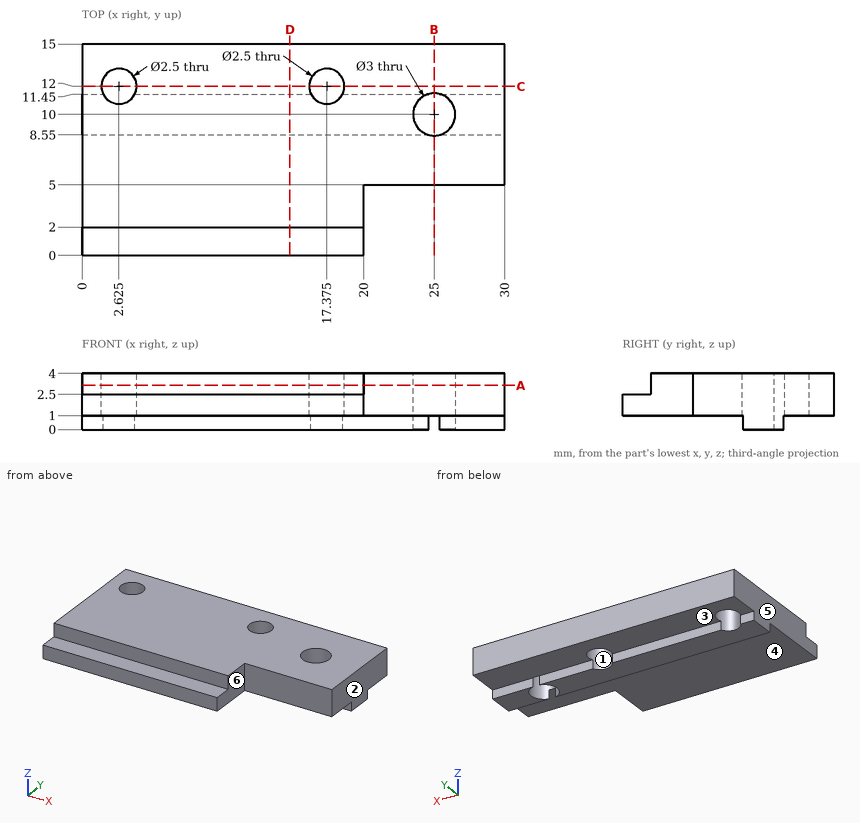
For this review, use the dimensioned drawing (mm, ordinates from the lowest corner) and the shaded views. A direction names the side the tool comes from. Give positions to 0.01 mm unless a question says otherwise; leave off trailing zeros. Loops run counter-clockwise (first coordinate to the right, second up) from the corner with the lowest first, then second, coordinate; pieces in that order, holes last.
Item 1: Insertion check: pin 1 (0.5 mm diameter, centred on x = 7.5, z = 0.5, fed in from +Y); pin 2 (0.8 mm diameter, centred on x = 1, z = 0.5, fed in from +Y); pin 3 (0.5 mm diameter, centred on x = 16.5, z = 0.5, fed in from -Y). Each pin has a flat end and moves straight along its axis. Give the tip position at first contact, or say it passes through.
Item 2: For line 1 along X through (y, z) = (12, 3.1) (3 decimals); line 2 along Y through (x, z) = (25, 2.15); line 3 along X through (y, z) = (10, 0.9), list the stretches that pass through material, from the lowest coordinate up.
Item 3: Take a section at B-B, the plane x = 25. State the section outline as (y, z) points.
Item 4: Take a section at C-C, the plane y = 12. State the section outline as (x, z) points (3 decimals).
Item 5: Take a section at A-A, the plane z = 3.15. State the section outline as (x, y) points (3 decimals).
Item 6: Tool access review of the marked faces 4, 5 and 6: name each direction out of +Z, -Z, +X, -X, +Y, -Y from which nothing blocks a thin tool from reaching the whole face with its end or side.
Item 7: Draft analysis for pull direction X (two halves, no side actions). For the marked faces 1, 2 and 3, state which applies: +X half, -X half, draft (parallel to the pull), parting line (faces both ways), or undercut.
Item 8: Take a section at D-D, the plane x = 14.75. State the section outline as (y, z) points, and give its area (3 significant figures).
Calculated:
1. pin 1: stops at y = 11.45
1. pin 2: stops at y = 11.45
1. pin 3: stops at y = 8.55
2. line 1: x = 0 to 1.375, 3.875 to 16.125, 18.625 to 30
2. line 2: y = 5 to 8.5, 11.5 to 15
2. line 3: x = 0 to 23.5, 26.5 to 30
3. outline: (5, 1) - (8.5, 1) - (8.5, 4) - (5, 4) - close; (11.5, 1) - (15, 1) - (15, 4) - (11.5, 4) - close
4. outline: (0, 1) - (1.375, 1) - (1.375, 4) - (0, 4) - close; (3.875, 1) - (16.125, 1) - (16.125, 4) - (3.875, 4) - close; (18.625, 1) - (30, 1) - (30, 4) - (18.625, 4) - close
5. outline: (0, 2) - (20, 2) - (20, 5) - (30, 5) - (30, 15) - (0, 15) - close; hole circle Ø2.5 at (2.625, 12); hole circle Ø2.5 at (17.375, 12); hole circle Ø3 at (25, 10)
6. face 4: -Z, +X, -X, -Y
6. face 5: +Z, -Z, -X, +Y, -Y
6. face 6: +Z, -Z, +X, -Y
7. face 1: undercut
7. face 2: +X half
7. face 3: draft
8. outline: (0, 1) - (8.55, 1) - (8.55, 0) - (11.45, 0) - (11.45, 1) - (15, 1) - (15, 4) - (2, 4) - (2, 2.5) - (0, 2.5) - close
8. area: 44.9 mm2
